Could you check a few things on this model? Use its own coordinates, in mm. A direction names the side the tool comes from. Coordinates: 2 decimals unless noted, no trailing zeros. Order: outer loops, then holes, each group sorted by start corner. A loop starts at its lowest first (then second) coordinate and runs counter-clockwise, first axis right, second up. Notation, with made-up numbers: (22, -4.5) - (35, -4.5) arc R18 cw to (35, 30.5) - close; hole circle Ø11 at (2, 33.5). An arc over 180 degrees is marked (long way). One line per item, written item: value. Start each with the question number.
Autodesk Inventor part; units mm, degrees
ref_plane "YZ Plane" through (0, 0, 0) normal (1, 0, 0) x (0, 1, 0)
ref_plane "XZ Plane" through (0, 0, 0) normal (0, 1, 0) x (-1, 0, 0)
ref_plane "XY Plane" through (0, 0, 0) normal (0, 0, 1) x (1, 0, 0)
sketch "Sketch1" plane through (0, 0, 0) normal (0, 0, 1) x (1, 0, 0)
  line L0 (11, 0) -> (22.5, 0)
  line L1 (11, 0) -> (11, 12)
  line L2 (11, 12) -> (19, 12)
  line L3 (32.5, 42) -> (22.5, 0)
  line L4 (19, 12) -> (26.1429, 42)
  line L5 (26.1429, 42) -> (32.5, 42)
  line L6 (0, -8.4) -> (0, 50.4)
  point P0 (0, 0)
  dimension "d0" = 11.5
  dimension "d1" = 11
  dimension "d2" = 22.5
  dimension "d3" = 12
  dimension "d4" = 19
  dimension "d5" = 8
  dimension "d7" = 6.1843
  dimension "d8" = 32.5
  dimension "d9" = 42
revolve "Revolution1" add sketch "Sketch1" angle 360 about axis through (0, -10, 0) along (0, 1, 0)
sketch "Sketch2" plane through (0, 0, 0) normal (0, 0, 1) x (1, 0, 0)
  line L0 (-32.5, 42) -> (32.5, 42)
  circle A0 centre (0, 42) radius 5
  point P0 (0, 0)
  dimension "d11" = 10
extrude "Extrusion1" cut sketch "Sketch2" along normal through all both and the other way through all
sketch "Sketch3" plane through (0, 0, 0) normal (1, 0, 0) x (0, 1, 0)
  line L0 (42, 25.6603) -> (42, -25.6603)
  circle A0 centre (42, 0) radius 5
  point P0 (0, 0)
  dimension "d14" = 10
extrude "Extrusion2" cut sketch "Sketch3" along normal through all both and the other way through all
properties part number "Screw Jack Cup"
Q1. I want a section at D-D on y = 28. Please give me the cut outline in (x, z), then the cut area to 3 significant figures.
Q2. Which directions (+Z, -Z, +X, -X, +Y, -Y) give clear straight access to the entire face, cutting with the end or side of a thin tool? Please do faces 5 (the flat face through (8, 12, 8)), 6 (the cylindrical face through (0, 37, 28)).
Q3. I'm going to push flat-ended pins straight in: pin 1 (4 mm diameter, centred on y = 29.5, z = -22.5, fed in from +X); pin 2 (1 mm diameter, centred on x = -3.5, y = 14, fed in from +Z); pin 3 (2 mm diameter, centred on x = 13, y = 8.5, fed in from +Z). Where does each tip first touch, or does it pass through?
Q4. We'd pull the mould along Z, two halves only. Please class faces 1 (the cylindrical face through (-2.38, 6.08, 10.74)), 2 (the conical face through (24.441, 16.627, 10.134)), 3 (the cylindrical face through (29, 37, 0)), 4 (the flat face through (19, 42, -19)): +Z half, -Z half, draft (parallel to the pull), parting line (faces both ways), or undercut.
Q5. I want a section at A-A on x = 0. Please give me the cut outline in (y, z).
Q6. If I drill on L1, parallel to Y at x = 5.5, z = 18; L2, parallel to X at y = 19.5, z = -14; L3, parallel to X at y = 11.5, z = 7.5, over which ranges is the centre line in solid material (lowest first)?
Q7. I want a section at B-B on z = 0. Please give me the cut outline in (x, y).
Q8. I want a section at C-C on y = 8.5. Please give me the cut outline in (x, z), then the cut area to 3 significant figures.
Values follow:
1. outline: circle Ø58.33 at (0, 0); hole circle Ø45.62 at (0, 0)
1. area: 1,040 mm^2
2. face 5: +Y
2. face 6: +Z, -Z, +Y
3. pin 1: stops at x = 21.36
3. pin 2: stops at z = 25.73
3. pin 3: stops at z = 21.45
4. face 1: undercut
4. face 2: parting line
4. face 3: undercut
4. face 4: draft
5. outline: (0, -22.5) - (37, -31.31) - (37, -24.95) - (12, -19) - (12, -11) - (0, -11) - close; (0, 11) - (12, 11) - (12, 19) - (37, 24.95) - (37, 31.31) - (0, 22.5) - close
6. L1: y = 0 to 12
6. L2: x = -23.25 to -15.36, 15.36 to 23.25
6. L3: x = -24.1 to -8.05, 8.05 to 24.1
7. outline: (-31.31, 37) - (-22.5, 0) - (-11, 0) - (-11, 12) - (-19, 12) - (-24.95, 37) - close; (11, 0) - (22.5, 0) - (31.31, 37) - (24.95, 37) - (19, 12) - (11, 12) - close
8. outline: circle Ø49.05 at (0, 0); hole circle Ø22 at (0, 0)
8. area: 1,510 mm^2
